Build history of the part. All positions in model axes, mm. Face numbers are marked on the shaded views. A direction names the side the tool comes from. Give positions to 0.01 mm unless a question says otherwise; leave off trailing zeros. Order: outer loops, then holes, each group sorted by start corner. A loop starts at its lowest first (then second) coordinate and runs counter-clockwise, first axis right, second up. Notation, with made-up numbers: (49.5, -34.75) - (94.5, -34.75) arc R18 ccw to (94.5, -16.75) - close; hole circle Ø4 at (58, 38.25). An arc over 180 degrees is marked (long way). Answer in a Markdown table with one row per item.
```python
from build123d import *

# Parameters (mm, degrees)
F0_W     = 44.083602
F0_H     = 33.323038
F1_DEPTH = 0.254
F2_W     = 44.083606
F2_H     = 24.686816
F3_DEPTH = 0.254
F4_W     = 44.083606
F4_H     = 25.171924
F5_DEPTH = 0.254
F6_W     = 43.984536
F6_H     = 17.969414
F7_DEPTH = 0.254
F8_W     = 43.022267
F8_H     = 15.82749
F9_DEPTH = 0.254


with BuildPart() as f1:
    # F0 (on Front) → F1 (new body)
    with BuildSketch(Plane.XZ):
        with Locations((0, -16.661519)):
            Rectangle(F0_W, F0_H)
    extrude(amount=F1_DEPTH)

    # F2 (on face) → F3 (join)
    with BuildSketch(Plane.XY):
        Rectangle(F2_W, F2_H)
    extrude(amount=F3_DEPTH)

    # F4 (on Front) → F5 (join)
    with BuildSketch(Plane.XZ):
        with Locations((0, 12.585962)):
            Rectangle(F4_W, F4_H)
    extrude(amount=F5_DEPTH)

    # F6 (on face) → F7 (join)
    with BuildSketch(Plane.XY.offset(25.171924)):
        Rectangle(F6_W, F6_H)
    extrude(amount=F7_DEPTH)

    # F8 (on Front) → F9 (join)
    with BuildSketch(Plane.XZ):
        with Locations((-0.362341, 32.440369)):
            Rectangle(F8_W, F8_H)
    extrude(amount=F9_DEPTH)


solid = f1.part
```
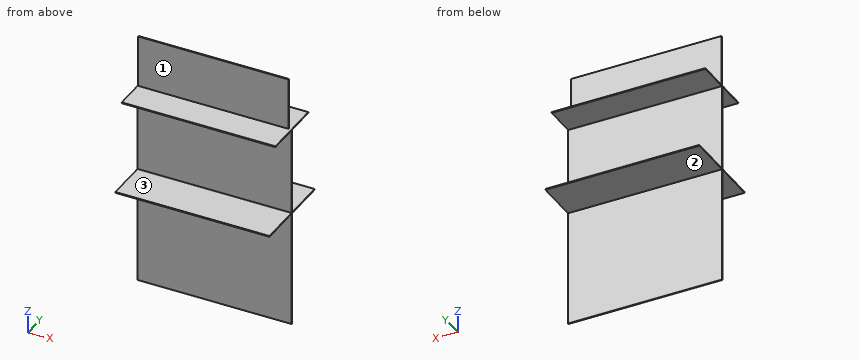
1. Probe line 1 (Z direction, x = -6, y = -5.25); line 2 (Y direction, x = 11, z = -10.5); line 3 (Z direction, x = -10.5, y = 9.75). List the from-to ranges inside material, lowest first.
Check result:
| item | result |
|---|---|
| line 1 | z = 0 to 0.25, 25.17 to 25.43 |
| line 2 | y = -0.25 to 0 |
| line 3 | z = 0 to 0.25 |
2. Cut at B-B on x = 5.5. Write the cut outline in (y, z).
Check result:
| item | result |
|---|---|
| outline | (-12.34, 0) - (-0.25, 0) - (-0.25, -33.32) - (0, -33.32) - (0, 0) - (12.34, 0) - (12.34, 0.25) - (0, 0.25) - (0, 25.17) - (8.98, 25.17) - (8.98, 25.43) - (0, 25.43) - (0, 40.35) - (-0.25, 40.35) - (-0.25, 25.43) - (-8.98, 25.43) - (-8.98, 25.17) - (-0.25, 25.17) - (-0.25, 0.25) - (-12.34, 0.25) - close |
3. Cut at C-C on z = -25. Write the cut outline in (x, y).
Check result:
| item | result |
|---|---|
| outline | (-22.04, -0.25) - (22.04, -0.25) - (22.04, 0) - (-22.04, 0) - close |
4. Cut at A-A on y = -2.75. Write the cut outline in (x, z).
Check result:
| item | result |
|---|---|
| outline | (-22.04, 0) - (22.04, 0) - (22.04, 0.25) - (-22.04, 0.25) - close; (-21.99, 25.17) - (21.99, 25.17) - (21.99, 25.43) - (-21.99, 25.43) - close |
5. Drop flat-ended pins along their axis: P1, Ø20, axis at x = 6.5, z = 14, coming from the -Y side; P2, Ø12, axis at x = -15, z = 10, coming from the +Y side; P3, Ø10, axis at x = -14, z = 4, coming from the +Y side; P4, Ø4.5, axis at x = 4, y = -7, coming from the -Z side. Give the stop position or say it passes through.
Check result:
| item | result |
|---|---|
| P1 | stops at y = -0.25 |
| P2 | stops at y = 0 |
| P3 | stops at y = 12.34 |
| P4 | stops at z = 0 |
6. Cut at D-D on y = 10.75. Write the cut outline in (x, z), and give its area (3 significant figures).
Check result:
| item | result |
|---|---|
| outline | (-22.04, 0) - (22.04, 0) - (22.04, 0.25) - (-22.04, 0.25) - close |
| area | 11.2 mm² |
7. Which spindle directions (+Z, -Z, +X, -X, +Y, -Y) get a long thin tool onto all of the face, cutting with end or side? Do the marked faces 1, 2 and 3. Say none if no direction does.
Check result:
| item | result |
|---|---|
| face 1 | +Z, +X, -X, -Y |
| face 2 | -Z, +X, -X, +Y |
| face 3 | +X, -X, -Y |
